Input: part model. Units: mm. Frame: model coordinates. Give positions to 0.01 mm unless a question says otherwise; leave off trailing zeros. Loops run counter-clockwise (first coordinate to the right, second up) from the corner with the lowest first, then second, coordinate; pieces in that order, holes last. Notation, with made-up numbers: (82.25, 14) -> (130.25, 14) arc R26 ccw to (130.25, 38) -> close; hole circle Ø10 at (7.25, 70.5). An arc over 180 degrees is marked (long way). Use CSV: the item, a comma, the result in double quotes.
```python
from build123d import *

# Parameters (mm, degrees)
SKETCH1_W           = 145
SKETCH1_H           = 60
BOSS_EXTRUDE1_DEPTH = 0.6
FILLET1_R           = 3
SKETCH2_R           = 1.35
CUT_EXTRUDE1_DEPTH  = 79.46406821


with BuildPart() as part:
    # Sketch1 → Boss-Extrude1 (new body)
    with BuildSketch(Plane.XY):
        Rectangle(SKETCH1_W, SKETCH1_H)
    extrude(amount=BOSS_EXTRUDE1_DEPTH)

    # Fillet1
    fillet1_edges = [part.edges().sort_by_distance(p)[0] for p in [
        (72.5, -30, 0.3),
        (-72.5, -30, 0.3),
        (-72.5, 30, 0.3),
        (72.5, 30, 0.3),
    ]]
    fillet(fillet1_edges, radius=FILLET1_R)

    # Sketch2 → Cut-Extrude1 (cut, through all)
    with BuildSketch(Plane.XY.offset(0.6)):
        with Locations((60, -27.5)):
            Circle(SKETCH2_R)
        with Locations((42.857142857, -27.5)):
            Circle(SKETCH2_R)
        with Locations((25.714285714, -27.5)):
            Circle(SKETCH2_R)
        with Locations((8.571428571, -27.5)):
            Circle(SKETCH2_R)
        with Locations((-8.571428571, -27.5)):
            Circle(SKETCH2_R)
        with Locations((-25.714285714, -27.5)):
            Circle(SKETCH2_R)
        with Locations((-42.857142857, -27.5)):
            Circle(SKETCH2_R)
        with Locations((-60, -27.5)):
            Circle(SKETCH2_R)
        with Locations((-70, -27.5)):
            Circle(SKETCH2_R)
        with Locations((-70, -17.5)):
            Circle(SKETCH2_R)
        with Locations((-70, -5.833333333)):
            Circle(SKETCH2_R)
        with Locations((-70, 5.833333333)):
            Circle(SKETCH2_R)
        with Locations((-70, 17.5)):
            Circle(SKETCH2_R)
        with Locations((-70, 27.5)):
            Circle(SKETCH2_R)
        with Locations((-60, 27.5)):
            Circle(SKETCH2_R)
        with Locations((-42.857142857, 27.5)):
            Circle(SKETCH2_R)
        with Locations((-25.714285714, 27.5)):
            Circle(SKETCH2_R)
        with Locations((-8.571428571, 27.5)):
            Circle(SKETCH2_R)
        with Locations((8.571428571, 27.5)):
            Circle(SKETCH2_R)
        with Locations((25.714285714, 27.5)):
            Circle(SKETCH2_R)
        with Locations((42.857142857, 27.5)):
            Circle(SKETCH2_R)
        with Locations((60, 27.5)):
            Circle(SKETCH2_R)
        with Locations((70, -27.5)):
            Circle(SKETCH2_R)
        with Locations((70, -17.5)):
            Circle(SKETCH2_R)
        with Locations((70, -5.833333333)):
            Circle(SKETCH2_R)
        with Locations((70, 5.833333333)):
            Circle(SKETCH2_R)
        with Locations((70, 17.5)):
            Circle(SKETCH2_R)
        with Locations((70, 27.5)):
            Circle(SKETCH2_R)
    extrude(amount=-CUT_EXTRUDE1_DEPTH, mode=Mode.SUBTRACT)


solid = part.part
```
1) Section query B-B (z = 0.3). Give the number of separate pieces and of enclosed holes in the cut face, then the cut area to 3 significant figures.
From the geometry:
separate pieces,"1"
enclosed holes,"28"
area,"8,530 mm^2"
2) Mould query, pull axis X, two halves, no side actions, for faces 1 (the flat face through (-1, 0, 0.6)), 2 (the cylindrical face through (-68.753, -18.017, 0.304)), 3 (the cylindrical face through (-71.64, -29.1, 0.3)), 4 (the cylindrical face through (71.247, -6.35, 0.304)). Classes: pulls with the +X half, pulls with the -X half, needs draft (parallel to the pull), parting line crosses it, or undercut.
From the geometry:
face 1,"needs draft"
face 2,"undercut"
face 3,"pulls with the -X half"
face 4,"undercut"
3) Section query A-A (x = -60). Return loops of the section in (y, z).
From the geometry:
outline,"(-30, 0) -> (-28.85, 0) -> (-28.85, 0.6) -> (-30, 0.6) -> close; (-26.15, 0) -> (26.15, 0) -> (26.15, 0.6) -> (-26.15, 0.6) -> close; (28.85, 0) -> (30, 0) -> (30, 0.6) -> (28.85, 0.6) -> close"
4) Ray query, line 1 (Y direction, x = 60, z = 0.3); line 2 (Y direction, x = -25, z = 0.25). Return the intervals inside material, ascending.
From the geometry:
line 1,"y = -30 to -28.85, -26.15 to 26.15, 28.85 to 30"
line 2,"y = -30 to -28.65, -26.35 to 26.35, 28.65 to 30"
